Can you work these out from the drawing? Everything is in mm from the part's minimum corner. A direction names the side the tool comes from. Coordinates: 2 decimals unless noted, no trailing zeros. Order: outer loops, then holes, each group sorted by start corner. A loop starts at its lowest first (then second) coordinate and runs counter-clockwise, first axis right, second up. Notation, with made-up numbers: (12, 82) - (54, 82) arc R30 cw to (54, 104) - close; hole circle Ø1 at (27.25, 38). An arc over 180 degrees is marked (long way). Use a Markdown table: item, result. Add a question column.
(1) On a 3-axis mill with a long thin cutter (end or side, diameter ignored), from which of +Z, -Z, +X, -X, +Y, -Y can I reach the whole of each face in a straight line? I mean the marked faces 1 and 2. Say none if no direction works.
(2) I want a section at C-C (y = 42.5). List the corners of the cut face in (x, z) for me, and give its area (3 significant figures).
(3) I want a section at A-A (x = 17). List the corners of the cut face in (y, z) for me.
(4) If I drill on L1, parallel to Z at x = 23, y = 37; L2, parallel to Y at x = 22.5, z = 2, over which ranges is the centre line in solid material (lowest first)? Write a range as [from, to].
(5) I want a section at B-B (z = 22). List the corners of the cut face in (x, y) for me, and give its area (3 significant figures).
(6) For pin 1 Ø5 at (x, z) = (34.5, 6.5) entering from +Y; pin 2 Ø20.5 at (x, y) = (31, 40) entering from -Z, each with a flat end and sliding along its axis, tell me the tip position at first contact or that it passes through.
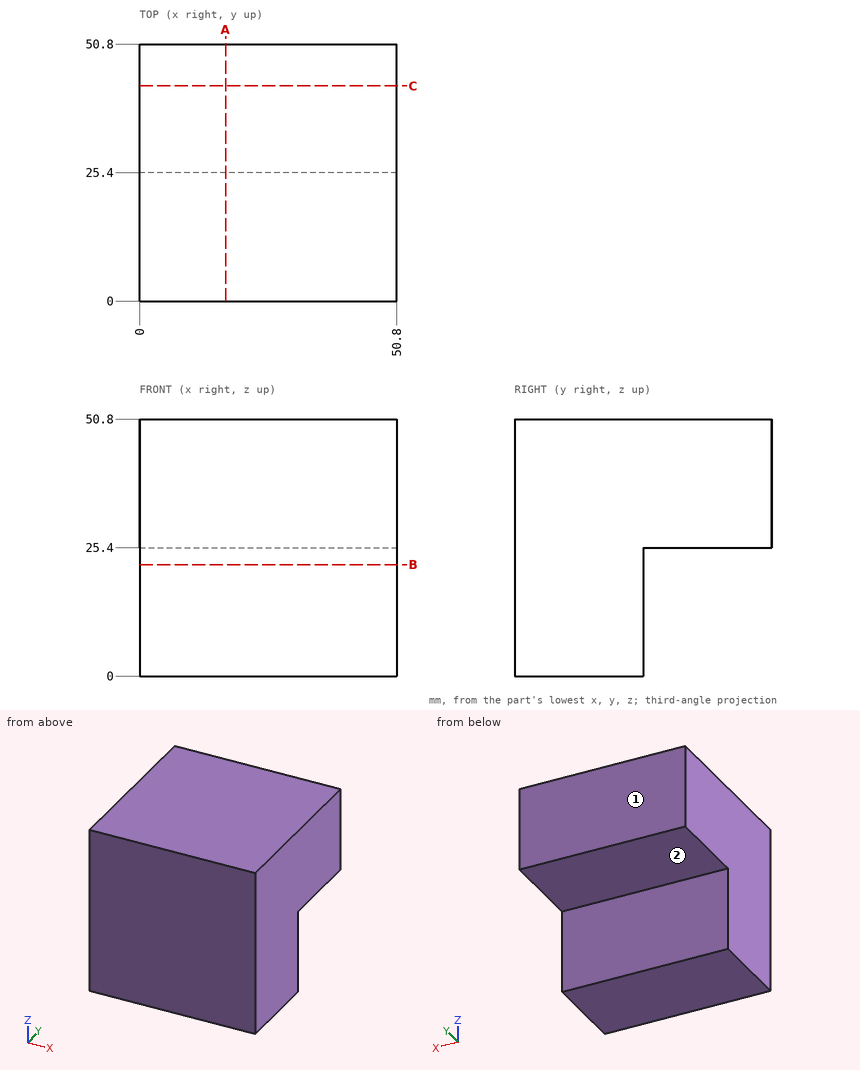
Answers follow:
| question | item | result |
|---|---|---|
| 1 | face 1 | +Z, -Z, +X, -X, +Y |
| 1 | face 2 | -Z, +X, -X, +Y |
| 2 | outline | (0, 25.4) - (50.8, 25.4) - (50.8, 50.8) - (0, 50.8) - close |
| 2 | area | 1,290 mm² |
| 3 | outline | (0, 0) - (25.4, 0) - (25.4, 25.4) - (50.8, 25.4) - (50.8, 50.8) - (0, 50.8) - close |
| 4 | L1 | z = [25.4, 50.8] |
| 4 | L2 | y = [0, 25.4] |
| 5 | outline | (0, 0) - (50.8, 0) - (50.8, 25.4) - (0, 25.4) - close |
| 5 | area | 1,290 mm² |
| 6 | pin 1 | stops at y = 25.4 |
| 6 | pin 2 | stops at z = 25.4 |
